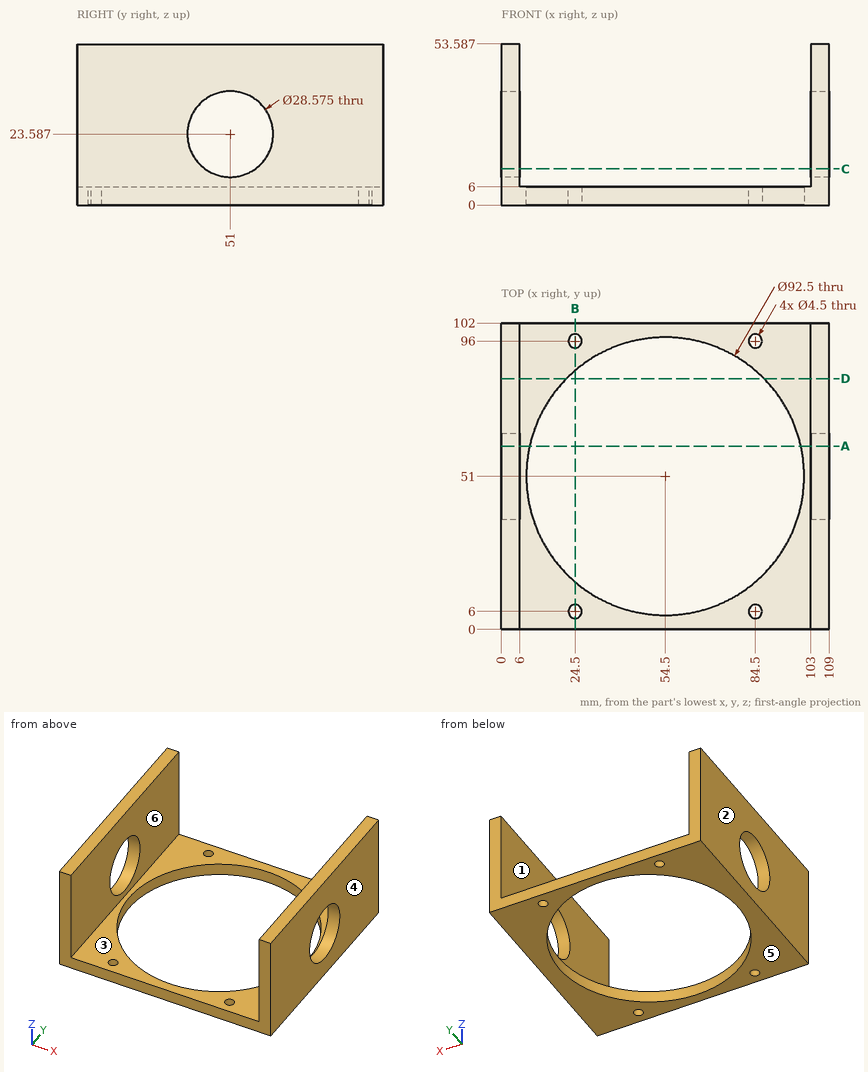
Design review of the part shown in the three views and the two pictorial views. Dimensions are in mm from the part's minimum x, y and z. A direction names the side the tool comes from. Round coordinates to 2 decimals unless told otherwise and drop trailing zeros. Loops run counter-clockwise (first coordinate to the right, second up) from the corner with the lowest first, then second, coordinate; pieces in that order, holes last.
Q1. Mouldability with a two-part tool opening along X and no side actions: class the marked faces 3, 4, 5 and 6 as +X half, -X half, draft (parallel to the pull), parting line (faces both ways), or undercut.
Result sheet:
face 3: undercut
face 4: +X half
face 5: draft
face 6: undercut
Q2. To check wall thickness, follow line 1 along X through (y, z) = (89, 44.5); line 2 along Y through (x, z) = (24, 2) (1 decimal); line 3 along Y through (x, z) = (24.5, 4.4). State the ranges of each line that lie inside material, in increasing order.
Result sheet:
line 1: x = 0 to 6, 103 to 109
line 2: y = 0 to 3.8, 8.2 to 16.2, 85.8 to 93.8, 98.2 to 102
line 3: y = 0 to 3.75, 8.25 to 15.8, 86.2 to 93.75, 98.25 to 102
Q3. Add section B-B on x = 24.5. Write out the cut boundary in (y, z).
Result sheet:
outline: (0, 0) - (3.75, 0) - (3.75, 6) - (0, 6) - close; (8.25, 0) - (15.8, 0) - (15.8, 6) - (8.25, 6) - close; (86.2, 0) - (93.75, 0) - (93.75, 6) - (86.2, 6) - close; (98.25, 0) - (102, 0) - (102, 6) - (98.25, 6) - close
Q4. Add section A-A on y = 61. Write out the cut boundary in (x, z) (1 decimal).
Result sheet:
outline: (0, 0) - (9.3, 0) - (9.3, 6) - (6, 6) - (6, 13.4) - (0, 13.4) - close; (0, 33.8) - (6, 33.8) - (6, 53.6) - (0, 53.6) - close; (99.7, 0) - (109, 0) - (109, 13.4) - (103, 13.4) - (103, 6) - (99.7, 6) - close; (103, 33.8) - (109, 33.8) - (109, 53.6) - (103, 53.6) - close
Q5. Machinability: for the marked faces 1 and 2, which of the approach directions +Z, -Z, +X, -X, +Y, -Y give a long, thin tool a straight path to every point of the face, cutting with its end or side? Answer none if there is none.
Result sheet:
face 1: +Z, +Y, -Y
face 2: +Z, -Z, -X, +Y, -Y
Q6. Add section D-D on y = 83.5. Write out the cut boundary in (x, z), plus the area to 3 significant figures.
Result sheet:
outline: (0, 0) - (21.59, 0) - (21.59, 6) - (6, 6) - (6, 53.59) - (0, 53.59) - close; (87.41, 0) - (109, 0) - (109, 53.59) - (103, 53.59) - (103, 6) - (87.41, 6) - close
area: 830 mm2
Q7. Add section C-C on z = 12. Write out the cut boundary in (x, y), plus the area to 3 significant figures.
Result sheet:
outline: (0, 0) - (6, 0) - (6, 42.64) - (0, 42.64) - close; (0, 59.36) - (6, 59.36) - (6, 102) - (0, 102) - close; (103, 0) - (109, 0) - (109, 42.64) - (103, 42.64) - close; (103, 59.36) - (109, 59.36) - (109, 102) - (103, 102) - close
area: 1,020 mm2
